Autodesk Inventor part; units mm, degrees
ref_plane "YZ Plane" through (0, 0, 0) normal (1, 0, 0) x (0, 1, 0)
ref_plane "XZ Plane" through (0, 0, 0) normal (0, 1, 0) x (-1, 0, 0)
ref_plane "XY Plane" through (0, 0, 0) normal (0, 0, 1) x (1, 0, 0)
sketch "Sketch1" plane through (0, 0, 0) normal (0, 1, 0) x (-1, 0, 0)
  line L0 (50.8, 342.9) -> (0, 342.9)
  line L1 (0, 342.9) -> (0, 292.1)
  line L2 (0, 292.1) -> (50.8, 292.1)
  line L3 (50.8, 292.1) -> (50.8, 342.9)
  line L4 (50.8, -292.1) -> (0, -292.1)
  line L5 (0, -292.1) -> (0, -241.3)
  line L6 (0, -241.3) -> (50.8, -241.3)
  line L7 (50.8, -241.3) -> (50.8, -292.1)
  line L8 (0, 0) -> (-42.6013, 0)
  dimension "d0" = 50.8
  dimension "d10" = 533.4
extrude "Extrusion1" add sketch "Sketch1" along normal blind 76.2
sketch "Sketch2" plane through (0, 0, 342.9) normal (1, 0, 0) x (0, 0, -1)
  line L0 (0, 76.2) -> (50.8, 76.2)
  line L1 (635, 0) -> (635, 76.2)
  line L2 (0, 76.2) -> (635, 76.2)
  line L3 (635, 76.2) -> (635, 50.8)
  line L4 (635, 50.8) -> (0, 50.8)
  line L5 (0, 50.8) -> (0, 76.2)
  point P0 (342.9, 0)
  dimension "d4" = 25.4
extrude "Extrusion2" add sketch "Sketch2" along normal blind 3.175
sketch "Sketch3" plane through (-50.8, 0, 292.1) normal (-1, 0, 0) x (0, 0, 1)
  line L0 (50.8, 76.2) -> (-584.2, 76.2)
  line L1 (-584.2, 76.2) -> (-584.2, 50.8)
  line L2 (-584.2, 50.8) -> (50.8, 50.8)
  line L3 (50.8, 50.8) -> (50.8, 76.2)
  line L4 (-533.4, 50.8) -> (0, 50.8)
  point P0 (-292.1, 0)
  dimension "d11" = 635
extrude "Extrusion3" add sketch "Sketch3" along normal blind 3.175
properties part number "crossbeam"
For this review, take the finished solid that the model builds, in its own axes (mm). A direction names the side the tool comes from. Coordinates: 2 decimals unless noted, no trailing zeros. Write each loop counter-clockwise with the first axis right and the second up, starting at its lowest first coordinate (ties: lowest second). Pieces come first, ordered by that corner, then holes. Notation, with made-up numbers: (-24.5, -23) - (-9.5, -23) arc R30 ccw to (-9.5, 14) - close; hole circle Ø7 at (-32.5, 19). An arc over 180 degrees is marked (long way). Answer in a Markdown table with one row per item. Add a question column.
Q1. Draft analysis for pull direction X (two halves, no side actions). For faces 6 (the flat face through (3.175, 64, 30)), 7 (the flat face through (0, 64, 29)), 8 (the flat face through (-25, 0, -266)), 9 (the flat face through (-25, 38, 292.1)), state which applies: +X half, -X half, draft (parallel to the pull), parting line (faces both ways), or undercut.
Q2. For P1, Ø15, axis at y = 18.5, z = 318, coming from the -X side; P2, Ø1.6, axis at x = 1, z = 33, coming from the -Y side, all flat-tipped, find the tip position at first contact; note any pin that passes through.
Q3. We need section B-B, the plane y = 11.5. State the section outline as (x, z) points, and give its area (3 significant figures).
Q4. For probe 1 along X at (y, z) = (71, 203) (3 decimals); probe 2 along Z at (x, y) = (-5.5, 4.5), list the stretches that pass through material, from the lowest coordinate up.
Q5. Tool access review of faces 1 (the flat face through (-53, 76.2, 27)), 2 (the flat face through (-50.8, 64, 22)), 3 (the flat face through (-50.8, 25, -266)), 4 (the flat face through (0, 25, 318)), 5 (the flat face through (-25, 39, -292.1)): name each direction out of +Z, -Z, +X, -X, +Y, -Y from which nothing blocks a thin tool from reaching the whole face with its end or side.
Q6. We need section A-A, the plane z = -168.5. State the section outline as (x, y) points (3 decimals).
Q7. We need section C-C, the plane y = 65.5. State the section outline as (x, z) points (3 decimals).
Answer list:
| question | item | result |
|---|---|---|
| 1 | face 6 | +X half |
| 1 | face 7 | undercut |
| 1 | face 8 | draft |
| 1 | face 9 | undercut |
| 2 | P1 | stops at x = -50.8 |
| 2 | P2 | stops at y = 50.8 |
| 3 | outline | (-50.8, -292.1) - (0, -292.1) - (0, -241.3) - (-50.8, -241.3) - close; (-50.8, 292.1) - (0, 292.1) - (0, 342.9) - (-50.8, 342.9) - close |
| 3 | area | 5,160 mm2 |
| 4 | probe 1 | x = -53.975 to -50.8, 0 to 3.175 |
| 4 | probe 2 | z = -292.1 to -241.3, 292.1 to 342.9 |
| 5 | face 1 | +Z, -Z, +X, -X, +Y |
| 5 | face 2 | +Y, -Y |
| 5 | face 3 | +Z, -Z, -X, -Y |
| 5 | face 4 | +Z, -Z, +X, -Y |
| 5 | face 5 | -Z, +X, -X, +Y, -Y |
| 6 | outline | (-53.975, 50.8) - (-50.8, 50.8) - (-50.8, 76.2) - (-53.975, 76.2) - close; (0, 50.8) - (3.175, 50.8) - (3.175, 76.2) - (0, 76.2) - close |
| 7 | outline | (-53.975, -292.1) - (3.175, -292.1) - (3.175, 342.9) - (-53.975, 342.9) - close; hole (-50.8, -241.3) - (0, -241.3) - (0, 292.1) - (-50.8, 292.1) - close |
